from build123d import *

# Parameters (mm, degrees)
F1_DEPTH = 6
F2_DEPTH = 2
F3_DEPTH = 1


# Not quite as in the source:
# - a feature names something its author has since deleted; it is built from what else it names


with BuildPart() as f1:
    # F0 (on Top) → F1 (new body)
    with BuildSketch(Plane.XY):
        with BuildLine():
            Line((-1.4142135624, 0.5), (1.4142135624, 0.5))
            ThreePointArc((1.4142135624, 0.5), (0, 1.5), (-1.4142135624, 0.5))
        make_face()
        with BuildLine():
            ThreePointArc((1.5, 0), (1.4783978395, 0.2536529681), (1.4142135624, 0.5))
            Line((1.4142135624, 0.5), (-1.4142135624, 0.5))
            ThreePointArc((-1.4142135624, 0.5), (-1.5, 0), (-1.4142135624, -0.5))
            Line((-1.4142135624, -0.5), (1.4142135624, -0.5))
            ThreePointArc((1.4142135624, -0.5), (1.4783978395, -0.2536529681), (1.5, 0))
        make_face()
        with BuildLine():
            ThreePointArc((-1.4142135624, -0.5), (0, -1.5), (1.4142135624, -0.5))
            Line((1.4142135624, -0.5), (-1.4142135624, -0.5))
        make_face()
    extrude(amount=-F1_DEPTH)

    # F0 (on Top) → F2 (join)
    with BuildSketch(Plane.XY):
        with BuildLine():
            ThreePointArc((-2.9580398915, -0.5), (0, -3), (2.9580398915, -0.5))
            Line((2.9580398915, -0.5), (1.4142135624, -0.5))
            ThreePointArc((1.4142135624, -0.5), (0, -1.5), (-1.4142135624, -0.5))
            Line((-1.4142135624, -0.5), (-2.9580398915, -0.5))
        make_face()
        with BuildLine():
            Line((1.4142135624, 0.5), (2.9580398915, 0.5))
            ThreePointArc((2.9580398915, 0.5), (0, 3), (-2.9580398915, 0.5))
            Line((-2.9580398915, 0.5), (-1.4142135624, 0.5))
            ThreePointArc((-1.4142135624, 0.5), (0, 1.5), (1.4142135624, 0.5))
        make_face()
        with BuildLine():
            Line((-1.4142135624, 0.5), (1.4142135624, 0.5))
            ThreePointArc((1.4142135624, 0.5), (0, 1.5), (-1.4142135624, 0.5))
        make_face()
        with BuildLine():
            ThreePointArc((-1.4142135624, -0.5), (0, -1.5), (1.4142135624, -0.5))
            Line((1.4142135624, -0.5), (-1.4142135624, -0.5))
        make_face()
    extrude(amount=F2_DEPTH)

    # F0 (on Top) → F3 (join)
    with BuildSketch(Plane.XY):
        with BuildLine():
            Line((-1.4142135624, 0.5), (-2.9580398915, 0.5))
            ThreePointArc((-2.9580398915, 0.5), (-3, 0), (-2.9580398915, -0.5))
            Line((-2.9580398915, -0.5), (-1.4142135624, -0.5))
            ThreePointArc((-1.4142135624, -0.5), (-1.5, 0), (-1.4142135624, 0.5))
        make_face()
        with BuildLine():
            ThreePointArc((1.5, 0), (1.4783978395, 0.2536529681), (1.4142135624, 0.5))
            Line((1.4142135624, 0.5), (-1.4142135624, 0.5))
            ThreePointArc((-1.4142135624, 0.5), (-1.5, 0), (-1.4142135624, -0.5))
            Line((-1.4142135624, -0.5), (1.4142135624, -0.5))
            ThreePointArc((1.4142135624, -0.5), (1.4783978395, -0.2536529681), (1.5, 0))
        make_face()
        with BuildLine():
            ThreePointArc((2.9580398915, -0.5), (2.9894915684, -0.2508787808), (3, 0))
            ThreePointArc((3, 0), (2.9894915684, 0.2508787808), (2.9580398915, 0.5))
            Line((2.9580398915, 0.5), (1.4142135624, 0.5))
            ThreePointArc((1.4142135624, 0.5), (1.4783978395, 0.2536529681), (1.5, 0))
            ThreePointArc((1.5, 0), (1.4783978395, -0.2536529681), (1.4142135624, -0.5))
            Line((1.4142135624, -0.5), (2.9580398915, -0.5))
        make_face()
    extrude(amount=F3_DEPTH)


solid = f1.part
Read the model definition and answer for the solid it produces. Units are mm, in the model's axes. A direction names the side the tool comes from. Coordinates: 2 decimals unless noted, no trailing zeros. Loops run counter-clockwise (first coordinate to the right, second up) from the corner with the lowest first, then second, coordinate; pieces in that order, holes last. Notation, with made-up numbers: (36.25, 20) -> (70.25, 20) arc R12 ccw to (70.25, 26) -> close; hole circle Ø11 at (19, 87.5). An arc over 180 degrees is marked (long way). Answer in a Markdown table with one row per item.
Item 1: For faces 1 (the flat face through (0, 0.5, 1.5)), 2 (the flat face through (0, 1, 2)), determine the directions among +Z, -Z, +X, -X, +Y, -Y from which every point of the face is accessible in a straight line to the end or side of a thin tool.
Returned:
| item | result |
|---|---|
| face 1 | +Z, +X, -X |
| face 2 | +Z, +X, -X, +Y, -Y |
Item 2: Each of these flat-tipped pins is pushed along its axis until it touches: P1, Ø3, axis at y = 1.5, z = -4.5, coming from the +X side; P2, Ø1, axis at x = -1, y = -2.5, coming from the -Z side; P3, Ø3, axis at x = 2, z = -4.5, coming from the +Y side. Where does it stop, or does it pass through?
Returned:
| item | result |
|---|---|
| P1 | stops at x = 1.5 |
| P2 | stops at z = 0 |
| P3 | stops at y = 1.41 |
Item 3: For a pull along Y with two mould halves and no side action, classify faces 3 (the flat face through (0, -0.5, 1.5)), 4 (the flat face through (1.3, -1.3, 0)) as released by +Y, released by -Y, zero draft, split by the parting line, or undercut.
Returned:
| item | result |
|---|---|
| face 3 | undercut |
| face 4 | zero draft |
Item 4: A cutting plane is placed at B-B on y = -2.4. Determine the outline of the cut face in (x, z).
Returned:
| item | result |
|---|---|
| outline | (-1.8, 0) -> (1.8, 0) -> (1.8, 2) -> (-1.8, 2) -> close |
Item 5: A cutting plane is placed at C-C on z = -2.75. Determine the outline of the cut face in (x, y).
Returned:
| item | result |
|---|---|
| outline | circle Ø3 at (0, 0) |
Item 6: Straight lines are drawn through the part: line 1 along Z through (x, y) = (0.05, -2.55); line 2 along Z through (x, y) = (-1.25, 0); line 3 along X through (y, z) = (-0.65, -0.5). For each, find the intervals that lie inside material, in ascending order. Write a range as [from, to].
Returned:
| item | result |
|---|---|
| line 1 | z = [0, 2] |
| line 2 | z = [-6, 1] |
| line 3 | x = [-1.35, 1.35] |
Item 7: A cutting plane is placed at D-D on x = 1.65. Determine the outline of the cut face in (y, z).
Returned:
| item | result |
|---|---|
| outline | (-2.51, 0) -> (2.51, 0) -> (2.51, 2) -> (0.5, 2) -> (0.5, 1) -> (-0.5, 1) -> (-0.5, 2) -> (-2.51, 2) -> close |
Item 8: A cutting plane is placed at A-A on x = -1.8. Determine the outline of the cut face in (y, z).
Returned:
| item | result |
|---|---|
| outline | (-2.4, 0) -> (2.4, 0) -> (2.4, 2) -> (0.5, 2) -> (0.5, 1) -> (-0.5, 1) -> (-0.5, 2) -> (-2.4, 2) -> close |
